Drawing for the job (mm, zero at the part's lowest x, y, z). A direction names the side the tool comes from. Give positions to 0.01 mm unless a question says otherwise; leave off trailing zeros. Order: outer loops, then holes, each group sorted by start corner. A loop starts at its lowest first (then second) coordinate and runs counter-clockwise, first axis right, second up. Notation, with made-up numbers: (1, 25) - (17, 25) arc R11 ccw to (17, 38) - close; hole circle Ø10 at (48, 57). An arc over 180 degrees is marked (long way). Use CSV: the item, a comma, the result in double quotes. Start each with the question number.
(1) Band-saw the part on A-A, the plane y = 4. Give the cut face in (x, z).
(2) Drop flat-ended pins along their axis: pin 1 Ø3 at (x, y) = (4, 4) entering from -Z; pin 2 Ø1.5 at (y, z) = (10, 3.5) entering from -X; pin 3 Ø1.5 at (y, z) = (15.5, 2) entering from +X. Give the stop position or say it passes through.
(3) Band-saw the part on D-D, the plane x = 56. Give the cut face in (y, z).
(4) Tool access for the marked faces 5, 6 and 7: list every direction of +Z, -Z, +X, -X, +Y, -Y with a clear straight run to the whole face (end or side of a thin tool).
(5) Band-saw the part on C-C, the plane z = 4.25. Give the cut face in (x, y), then the cut area to 3 significant figures.
(6) Probe L1, parallel to Y at x = 56, z = 1.45; L2, parallel to Y at x = 24, z = 1.75; L3, parallel to Y at x = 7, z = 2.35. List the from-to ranges inside material, lowest first.
(7) Band-saw the part on B-B, the plane x = 16.5. Give the cut face in (y, z).
(8) Pull direction Y, two halves, no side cores. Call the marked faces 1, 2, 3 and 4: +Y half, -Y half, draft (parallel to the pull), parting line (faces both ways), or undercut.
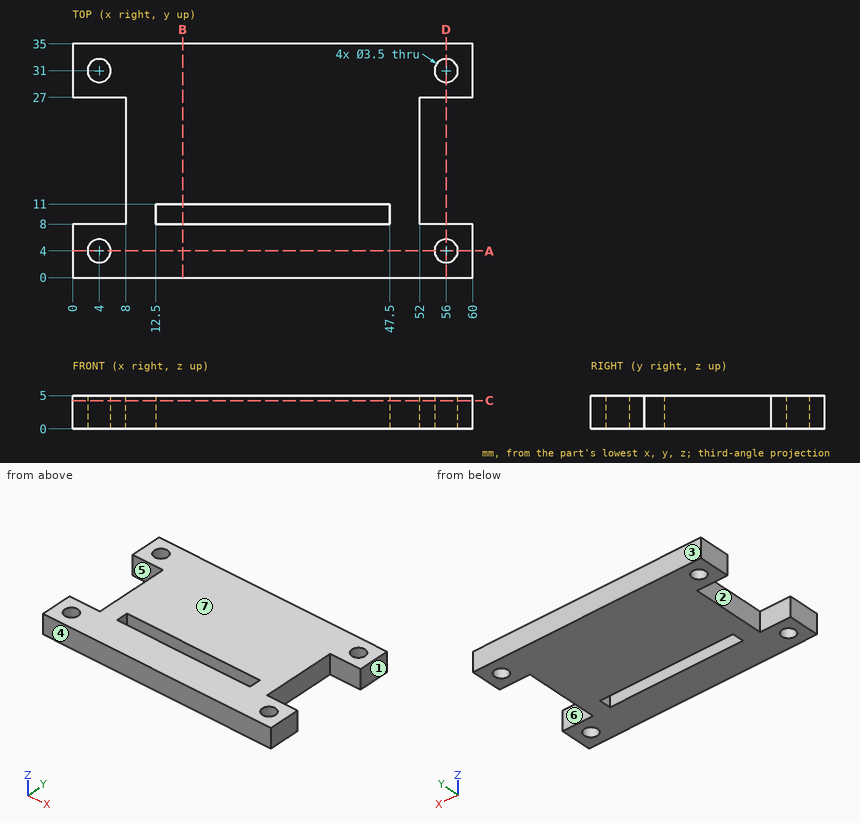
Answer block:
1,outline,"(0, 0) - (2.25, 0) - (2.25, 5) - (0, 5) - close; (5.75, 0) - (54.25, 0) - (54.25, 5) - (5.75, 5) - close; (57.75, 0) - (60, 0) - (60, 5) - (57.75, 5) - close"
2,pin 1,"passes through"
2,pin 2,"stops at x = 8"
2,pin 3,"stops at x = 52"
3,outline,"(0, 0) - (2.25, 0) - (2.25, 5) - (0, 5) - close; (5.75, 0) - (8, 0) - (8, 5) - (5.75, 5) - close; (27, 0) - (29.25, 0) - (29.25, 5) - (27, 5) - close; (32.75, 0) - (35, 0) - (35, 5) - (32.75, 5) - close"
4,face 5,"+Z, -Z, -X"
4,face 6,"+Z, -Z, +X"
4,face 7,"+Z, +X, -X, +Y, -Y"
5,outline,"(0, 0) - (60, 0) - (60, 8) - (52, 8) - (52, 27) - (60, 27) - (60, 35) - (0, 35) - (0, 27) - (8, 27) - (8, 8) - (0, 8) - close; hole circle Ø3.5 at (4, 4); hole circle Ø3.5 at (4, 31); hole (12.5, 8) - (47.5, 8) - (47.5, 11) - (12.5, 11) - close; hole circle Ø3.5 at (56, 4); hole circle Ø3.5 at (56, 31)"
5,area,"1,650 mm2"
6,L1,"y = 0 to 2.25, 5.75 to 8, 27 to 29.25, 32.75 to 35"
6,L2,"y = 0 to 8, 11 to 35"
6,L3,"y = 0 to 8, 27 to 35"
7,outline,"(0, 0) - (8, 0) - (8, 5) - (0, 5) - close; (11, 0) - (35, 0) - (35, 5) - (11, 5) - close"
8,face 1,"draft"
8,face 2,"undercut"
8,face 3,"+Y half"
8,face 4,"-Y half"
